Autodesk Inventor part; units mm, degrees
ref_plane "bolt_XY" through (0, 0, 0) normal (1, 0, 0) x (0, 0, -1)
ref_plane "bolt_YZ" through (0, 0, 0) normal (0, 0, -1) x (0, 1, 0)
ref_plane "bolt_ZX" through (0, 0, 0) normal (0, 1, 0) x (1, 0, 0)
sketch "Sketch_1" plane through (0, 0, 0) normal (0, 0, 1) x (1, 0, 0)
  line L0 (22, 0) -> (-5, 0)
  line L1 (-5, 0) -> (-5, 3.75)
  line L2 (-5, 3.75) -> (-4.5, 4.25)
  line L3 (-4.5, 4.25) -> (0, 4.25)
  line L4 (0, 4.25) -> (0, 2.5)
  line L5 (0, 2.5) -> (21.5095, 2.5)
  line L6 (21.5095, 2.5) -> (22, 2.0095)
  line L7 (22, 2.0095) -> (22, 0)
  line L8 (22, 0) -> (-5, 0)
revolve "Revolution1" add sketch "Sketch_1" angle 360 about axis through (22, 0, 0) along (1, 0, 0)
thread "Thread1"
sketch "Sketch2" plane through (-5, 0, 0) normal (-1, 0, 0) x (0, 0, 1)
  point P0 (0, 0)
hole "Hole1" at (-5, 0, 0) direction (1, 0, 0) diameter 4 depth 2.5 tip angle 150
sketch "Sketch_3" plane through (-5, 0, 0) normal (1, 0, 0) x (0, 0, -1)
  line L0 (-2, -1.1547) -> (0, -2.3094)
  line L1 (0, -2.3094) -> (2, -1.1547)
  line L2 (2, -1.1547) -> (2, 1.1547)
  line L3 (2, 1.1547) -> (0, 2.3094)
  line L4 (0, 2.3094) -> (-2, 1.1547)
  line L5 (-2, 1.1547) -> (-2, -1.1547)
extrude "Extrusion1" cut sketch "Sketch_3" along normal blind 2.5
ref_plane "bolt_XY" through (0, 0, 0) normal (1, 0, 0) x (0, 0, -1)
ref_plane "bolt_YZ" through (0, 0, 0) normal (0, 0, -1) x (0, 1, 0)
ref_plane "bolt_ZX" through (0, 0, 0) normal (0, 1, 0) x (1, 0, 0)
ref_plane "nut_XY" through (22, 0, 0) normal (1, 0, 0) x (0, 0, -1)
ref_plane "nut_YZ" through (22, 0, 0) normal (0, 0, -1) x (0, 1, 0)
ref_plane "nut_ZX" through (22, 0, 0) normal (0, 1, 0) x (1, 0, 0)
properties part number "SCB5-22"
Model file for the job. Use its own axes, mm. A direction names the side the tool comes from. Coordinates: 2 decimals unless noted, no trailing zeros. Write each loop counter-clockwise with the first axis right and the second up, starting at its lowest first coordinate (ties: lowest second). Pieces come first, ordered by that corner, then holes. Notation, with made-up numbers: (-38, 32.25) - (19, 32.25) arc R9 cw to (19, 37.25) - close; hole circle Ø6 at (22.5, 23.5). An arc over 180 degrees is marked (long way). Use a Markdown table: item, result. Add a question column.
Item 1: Drop flat-ended pins along their axis: pin 1 (4 mm diameter, centred on x = 11, z = -3, fed in from +Y); pin 2 (1.5 mm diameter, centred on x = 0.5, y = 1, fed in from -Z); pin 3 (1.5 mm diameter, centred on x = 2.5, z = 1.5, fed in from -Y); pin 4 (1.8 mm diameter, centred on x = -3, y = -0.5, fed in from +Z). Give the stop position or say it passes through.
Item 2: Two-plate mould, pull along Y, no slides. Class faces 3 (the face through (-1.998, -0.122, -0.027)), 4 (the face through (10.91, -0.54, -2.44)), 5 (the face through (0, 2, -2)), 6 (the face through (-3.77, -1.74, -0.99)): pulls with the +Y half, pulls with the -Y half, needs draft (parallel to the pull), parting line crosses it, or undercut.
Item 3: 3-axis set-ups, long thin cutter, end or side, ignore diameter. For faces 1 (the face through (22, 0, 0)), 2 (the face through (-4, 0, 2)): which of +Z, -Z, +X, -X, +Y, -Y reach the whole face in a straight line?
Item 4: Drill centre lines: line 1 along Z through (x, y) = (16.25, 1.5); line 2 along X through (y, z) = (1.75, -2.5). Where is each one in solid material? Low to high.
Item 5: Band-saw the part on A-A, the plane x = 3.5. Write the cut outline in (y, z), and give its area (3 significant figures).
A:
| question | item | result |
|---|---|---|
| 1 | pin 1 | stops at y = 2.29 |
| 1 | pin 2 | stops at z = -4.23 |
| 1 | pin 3 | stops at y = -2.38 |
| 1 | pin 4 | stops at z = 4.25 |
| 2 | face 3 | undercut |
| 2 | face 4 | parting line crosses it |
| 2 | face 5 | needs draft |
| 2 | face 6 | undercut |
| 3 | face 1 | +Z, -Z, +X, +Y, -Y |
| 3 | face 2 | -X |
| 4 | line 1 | z = -2 to 2 |
| 4 | line 2 | x = -5 to 0 |
| 5 | outline | circle Ø5 at (0, 0) |
| 5 | area | 19.6 mm² |
